The listing builds one solid part. Answer for the finished solid, in the listing's coordinates (mm). A direction names the side the tool comes from. Round coordinates to 2 decimals unless told otherwise and drop trailing zeros. Order: outer loops, then holes, each group sorted by start corner. A loop starts at its lowest first (then second) coordinate and runs counter-clockwise, first axis right, second up. Notation, with made-up numbers: (49, -1) -> (85, -1) arc R20 cw to (85, 10) -> close; hole circle Ø8 at (44, 77.5). An arc over 180 degrees is marked (long way). Return JSON: item names as keys, results as strings. Group by question number.
(1) The part is cut by section A-A (y = 0). Determine the outline of the cut face in (x, z).
(2) Consider line 1 (X direction, y = -2.5, z = -0.7); line 2 (X direction, y = -1.5, z = 0.8); line 3 (Z direction, x = 6.5, y = -0.5). Determine where each line is inside the solid, lowest interval first. Write a range as [from, to].
(3) Which of the six approach directions +Z, -Z, +X, -X, +Y, -Y give full straight-line access (tool end or side, diameter ignored) to faces 1 (the face through (-1.857, -1.46, 2.556)), 2 (the face through (3.8, -1.5, 0.07))?
(4) This flat-tipped pin is pushed along its axis until it touches: pin 1 (1 mm diameter, centred on y = -0.5, z = 2, fed in from +X). Where does it stop, or does it pass through?
(5) The part is cut by section B-B (x = 6). Determine the outline of the cut face in (y, z), plus the area to 3 significant figures.
from build123d import *

# Parameters (mm, degrees)
SKETCH2_OUTSIDE_W  = 11.336
SKETCH2_OUTSIDE_H  = 11.336
CUT_EXTRUDE1_DEPTH = 10


with BuildPart() as part:
    # Sketch1 → Revolve1 (revolve)
    with BuildSketch(Plane.XY):
        Polygon((0, 1.5), (0, 2.4), (-0.25, 2.4), (-0.25, 3.3), (-1.5, 3.3), (-2, 2.8), (-2, 0), (8, 0), (8, 1), (7.711324865, 1.5), align=None)
    revolve(axis=Axis((-88.99, 0, 0), (1, 0, 0)))

    # Sketch2 outside → Cut-Extrude1 (cut)
    with BuildSketch(Plane(origin=(0, 0, 0), x_dir=(0, 0, -1), z_dir=(1, 0, 0))):
        Rectangle(SKETCH2_OUTSIDE_W, SKETCH2_OUTSIDE_H)
        Polygon((0, 3.175426481), (-2.75, 1.58771324), (-2.75, -1.58771324), (0, -3.175426481), (2.75, -1.58771324), (2.75, 1.58771324), align=None, mode=Mode.SUBTRACT)
    extrude(amount=-CUT_EXTRUDE1_DEPTH, mode=Mode.SUBTRACT)


solid = part.part
Answer below:
{
 "1": {"outline": "(-2, -2.75) -> (-0.25, -2.75) -> (-0.25, -2.4) -> (0, -2.4) -> (0, -1.5) -> (7.71, -1.5) -> (8, -1) -> (8, 1) -> (7.71, 1.5) -> (0, 1.5) -> (0, 2.4) -> (-0.25, 2.4) -> (-0.25, 2.75) -> (-2, 2.75) -> close"},
 "2": {"line 1": "x = [-2, -0.25]", "line 2": "x = [-2, 0]", "line 3": "z = [-1.41, 1.41]"},
 "3": {"face 1": "+Z, -X, -Y", "face 2": "+X"},
 "4": {"pin 1": "stops at x = 0"},
 "5": {"outline": "circle Ø3 at (0, 0)", "area": "7.07 mm²"}
}
